Could you check a few things on this model? Use its own coordinates, in mm. Face numbers are marked on the shaded views. A direction names the side the tool comes from. Coordinates: 2 decimals unless noted, no trailing zeros. Order: outer loops, then holes, each group sorted by start corner. A loop starts at its lowest first (then second) coordinate and runs counter-clockwise, first axis right, second up. Notation, with made-up numbers: M 89,55 L 124,55 A23 cw 124,80 Z; hole C 59,1 d7. An arc over 180 degrees is marked long. Put each result on its own line as item: value. Start each with the question number.
```python
from build123d import *

# Parameters (mm, degrees)
ESBO_O1_R                = 4.5
RESSALTO_EXTRUS_O1_DEPTH = 28
CORTE_EXTRUS_O5_START    = 28
ESBO_O1_3_R              = 13.5
ESBO_O1_3_W              = 12.4
ESBO_O1_3_H              = 6
CORTE_EXTRUS_O5_DEPTH    = 54
ESBO_O3_R                = 1
CORTE_EXTRUS_O3_DEPTH    = 10
CORTE_EXTRUS_O4_DEPTH    = 2
ESBO_O5_R                = 1.65
CORTE_EXTRUS_O6_DEPTH    = 2.5
ESBO_O5_2_R              = 1.65
CORTE_EXTRUS_O7_DEPTH    = 6
ESBO_O6_W                = 5
ESBO_O6_H                = 3
CORTE_EXTRUS_O8_DEPTH    = 3


with BuildPart() as part:
    # Esboço1 → Ressalto-extrusão1 (new body, symmetric)
    with BuildSketch(Plane.XY):
        with BuildLine():
            Line((-16, 0), (-16, -25.5))
            Line((-16, -25.5), (10, -25.5))
            Line((10, -25.5), (10, -20.5))
            Line((10, -20.5), (0, -20.5))
            Line((0, -20.5), (0, -17.5))
            Line((0, -17.5), (10, -17.5))
            Line((10, -17.5), (10, -11.401754251))
            ThreePointArc((10, -11.401754251), (5.724949799, 14.195069567), (-16, 0))
        make_face()
        with Locations((-0.5, 0)):
            Circle(ESBO_O1_R, mode=Mode.SUBTRACT)
        with BuildLine():
            Line((-2.2, 8), (-2.2, 11))
            ThreePointArc((-2.2, 11), (-0.5, 12.7), (1.2, 11))
            Line((1.2, 11), (1.2, 8))
            ThreePointArc((1.2, 8), (-0.5, 6.3), (-2.2, 8))
        make_face(mode=Mode.SUBTRACT)
        with BuildLine():
            Line((-2.2, -8), (-2.2, -11))
            ThreePointArc((-2.2, -11), (-0.5, -12.7), (1.2, -11))
            Line((1.2, -11), (1.2, -8))
            ThreePointArc((1.2, -8), (-0.5, -6.3), (-2.2, -8))
        make_face(mode=Mode.SUBTRACT)
    extrude(amount=RESSALTO_EXTRUS_O1_DEPTH, both=True)

    # Esboço1<3> → Corte-extrusão5 (cut)
    with BuildSketch(Plane.XY.offset(CORTE_EXTRUS_O5_START)):
        with Locations((-0.5, 0)):
            Circle(ESBO_O1_3_R)
        with Locations((-8.2, -21)):
            Rectangle(ESBO_O1_3_W, ESBO_O1_3_H)
    extrude(amount=-CORTE_EXTRUS_O5_DEPTH, mode=Mode.SUBTRACT)

    # Esboço3 → Corte-extrusão3 (cut)
    with BuildSketch(Plane.XY.offset(28)):
        with Locations((-12, -12)):
            Circle(ESBO_O3_R)
        Polygon((-8, -11.22497216), (-8, -18), (-2, -18), (-2, -13.416407865), align=None)
    extrude(amount=-CORTE_EXTRUS_O3_DEPTH, mode=Mode.SUBTRACT)

    # Esboço4 → Corte-extrusão4 (cut)
    with BuildSketch(Plane.XY.offset(28)):
        with BuildLine():
            Line((-2, -25.5), (-16, -25.5))
            Line((-16, -25.5), (-16, 0))
            ThreePointArc((-16, 0), (5.724949799, 14.195069567), (10, -11.401754251))
            Line((10, -11.401754251), (10, -16))
            Line((10, -16), (-2, -16))
            Line((-2, -16), (-2, -25.5))
        make_face()
    extrude(amount=-CORTE_EXTRUS_O4_DEPTH, mode=Mode.SUBTRACT)

    # Esboço5 → Corte-extrusão6 (cut)
    with BuildSketch(Plane(origin=(0, -20.5, 0), x_dir=(1, 0, 0), z_dir=(0, 1, 0))):
        Polygon((5, 14.035898385), (8, 15.767949192), (8, 19.232050808), (5, 20.964101615), (2, 19.232050808), (2, 15.767949192), align=None)
        with Locations((5, 17.5)):
            Circle(ESBO_O5_R, mode=Mode.SUBTRACT)
        Polygon((5, -20.964101615), (8, -19.232050808), (8, -15.767949192), (5, -14.035898385), (2, -15.767949192), (2, -19.232050808), align=None)
        with Locations((5, -17.5)):
            Circle(ESBO_O5_R, mode=Mode.SUBTRACT)
    extrude(amount=-CORTE_EXTRUS_O6_DEPTH, mode=Mode.SUBTRACT)

    # Esboço5<2> → Corte-extrusão7 (cut, through all)
    with BuildSketch(Plane(origin=(0, -20.5, 0), x_dir=(1, 0, 0), z_dir=(0, 1, 0))):
        with Locations((5, -17.5)):
            Circle(ESBO_O5_2_R)
        with Locations((5, 17.5)):
            Circle(ESBO_O5_2_R)
    extrude(amount=-CORTE_EXTRUS_O7_DEPTH, mode=Mode.SUBTRACT)

    # Esboço6 → Corte-extrusão8 (cut, through all)
    with BuildSketch(Plane.XY.offset(-26)):
        with Locations((-11.9, -22.5)):
            Rectangle(ESBO_O6_W, ESBO_O6_H)
    extrude(amount=-CORTE_EXTRUS_O8_DEPTH, mode=Mode.SUBTRACT)


solid = part.part
```
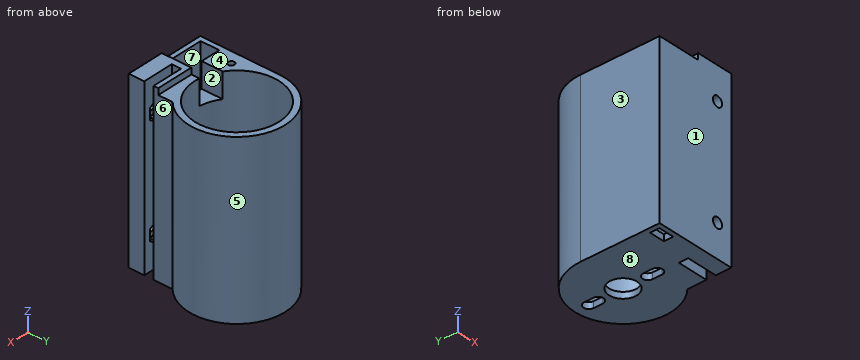
Item 1: For pin 1 Ø2 at (y, z) = (-22, -17.5) entering from +X; pin 2 Ø1 at (y, z) = (-5, -8) entering from +X; pin 3 Ø1 at (y, z) = (-10, -26.5) entering from +X; pin 4 Ø11 at (x, z) = (4.5, 10) entering from +Y, each with a flat end and sliding along its axis, tell me the tip position at first contact or that it passes through.
Item 2: I need wall thicknesses on probe 1 along Z at (x, y) = (5, -23.8); probe 2 along Y at (x, z) = (-0.5, -26.4); probe 3 along X at (y, z) = (0, -6.5). Which ranges of each line are inside material? Lowest first, please.
Item 3: If we mould it in two halves opening along X, with no side actions, what happens to the marked faces 1, 2 and 3? For each: released by +X, released by -X, zero draft, split by the parting line, or undercut.
Item 4: If we section it at B-B on z = -9.5: Write out the boundary of the cut face in (x, y).
Item 5: For the marked faces 4, 5, 6, 7 and 8, which set-ups out of +Z, -Z, +X, -X, +Y, -Y let a thin tool reach every point of the face, with its end or its side?
Item 6: If we section it at A-A on z = -17.5: Write out the boundary of the cut face in (x, y), then the cut area to 3 significant figures.
Geometry check:
1. pin 1: stops at x = 10
1. pin 2: stops at x = 14.33
1. pin 3: stops at x = 11.75
1. pin 4: stops at y = 15.5
2. probe 1: z = -28 to -19.15, -15.85 to 15.85, 19.15 to 28
2. probe 2: y = -25.5 to -12.7, -6.3 to -4.5, 4.5 to 6.3, 12.7 to 15.5
2. probe 3: x = -16 to -14, 13 to 15
3. face 1: zero draft
3. face 2: undercut
3. face 3: released by -X
4. outline: M -16,-25.5 L 10,-25.5 L 10,-20.5 L 0,-20.5 L 0,-17.5 L 10,-17.5 L 10,-11.4 A15.5 ccw long -16,0 Z; hole M -14.4,-24 L -2,-24 L -2,-18 L -14.4,-18 Z; hole C -0.5,0 d27
5. face 4: +Z, -X, +Y
5. face 5: +Z, -Z
5. face 6: +Z, -Z, +X, -Y
5. face 7: +Z
5. face 8: -Z, +X, -X, +Y, -Y
6. outline: M -16,-25.5 L 3.35,-25.5 L 3.35,-23 L 2,-23 L 2,-20.5 L 0,-20.5 L 0,-17.5 L 10,-17.5 L 10,-11.4 A15.5 ccw long -16,0 Z; M 6.65,-25.5 L 10,-25.5 L 10,-20.5 L 8,-20.5 L 8,-23 L 6.65,-23 Z; hole M -14.4,-24 L -2,-24 L -2,-18 L -14.4,-18 Z; hole C -0.5,0 d27
6. area: 380 mm²
